```python
from build123d import *

# Parameters (mm, degrees)
CUT_EXTRUDE_1_REACH = 18
SKETCH_2_R          = 1


with BuildPart() as part:
    # Эскиз1 → Повернуть1 (revolve)
    with BuildSketch(Plane.XY):
        Polygon((0, 0), (12.5, 0), (12.5, 4), (14.5, 4), (14.5, 15), (16, 15), (16, -1), (0, -1), align=None)
    revolve(axis=Axis((0, -1, 0), (0, 1, 0)))

    # Эскиз2 → Вырез-Вытянуть1 (cut, up to next)
    with BuildSketch(Plane.XY, mode=Mode.PRIVATE) as cut_extrude_1_sk1:
        with Locations((0, 8)):
            Circle(SKETCH_2_R)
    cut_extrude_1_tool1 = extrude(cut_extrude_1_sk1.sketch, amount=-CUT_EXTRUDE_1_REACH, mode=Mode.PRIVATE) & part.part
    add(cut_extrude_1_tool1.solids().sort_by_distance((0, 8, 0))[0], mode=Mode.SUBTRACT)


solid = part.part
```
The listing builds one solid part. Answer for the finished solid, in the listing's coordinates (mm). A direction names the side the tool comes from. Coordinates: 2 decimals unless noted, no trailing zeros. Write each loop counter-clockwise with the first axis right and the second up, starting at its lowest first coordinate (ties: lowest second). Pieces come first, ordered by that corner, then holes.
Q1. Which of the six approach directions +Z, -Z, +X, -X, +Y, -Y give full straight-line access (tool end or side, diameter ignored) to faces 1 (the flat face through (0, -1, 0)), 2 (the cylindrical face through (11.923, 2.028, -3.755))?
Returned:
face 1: +Z, -Z, +X, -X, -Y
face 2: +Y
Q2. Section B-B, the plane z = 0 is taken. Write down the section's boundary in (x, y).
Returned:
outline: (-16, -1) - (16, -1) - (16, 15) - (14.5, 15) - (14.5, 4) - (12.5, 4) - (12.5, 0) - (-12.5, 0) - (-12.5, 4) - (-14.5, 4) - (-14.5, 15) - (-16, 15) - close
Q3. Find the intervals of material crossed by line 1 along X through (y, z) = (1.95, 0); line 2 along X through (y, z) = (7, 0), in increasing order.
Returned:
line 1: x = -16 to -12.5, 12.5 to 16
line 2: x = -16 to -14.5, 14.5 to 16
Q4. Given P1, Ø1.8, axis at x = 0, y = 8, coming from the -Z side; P2, Ø1, axis at x = -8.5, z = 4, coming from the +Y side; P3, Ø1, axis at x = 1, y = 0.5, coming from the +Z side, each flat-ended and moving along its own axis, determine where each tip first touches the part or whether it passes through.
Returned:
P1: stops at z = 14.47
P2: stops at y = 0
P3: stops at z = 15.99
Q5. The mould has two halves that part along X. Classify faces 3 (the cylindrical face through (0, 9, -15)), 4 (the cylindrical face through (-3.47, 6.89, 15.62)), 5 (the flat face through (3.6, 15, -14.3)): released by +X, released by -X, zero draft, split by the parting line, or undercut.
Returned:
face 3: undercut
face 4: split by the parting line
face 5: zero draft
Q6. Section A-A, the plane x = 0 is taken. Write down the section's boundary in (y, z), then the cut area to 3 significant figures.
Returned:
outline: (-1, -16) - (7, -16) - (7, -14.5) - (4, -14.5) - (4, -12.5) - (0, -12.5) - (0, 12.5) - (4, 12.5) - (4, 14.5) - (15, 14.5) - (15, 16) - (-1, 16) - close; (9, -16) - (15, -16) - (15, -14.5) - (9, -14.5) - close
area: 90.0 mm2
Q7. Section C-C, the plane y = 1.5 is taken. Write down the section's boundary in (x, z), then the cut area to 3 significant figures.
Returned:
outline: circle Ø32 at (0, 0); hole circle Ø25 at (0, 0)
area: 313 mm2
Q8. Section D-D, the plane x = -10 is taken. Write down the section's boundary in (y, z), then the cut area to 3 significant figures.
Returned:
outline: (-1, -12.49) - (15, -12.49) - (15, -10.5) - (4, -10.5) - (4, -7.5) - (0, -7.5) - (0, 7.5) - (4, 7.5) - (4, 10.5) - (15, 10.5) - (15, 12.49) - (-1, 12.49) - close
area: 109 mm2
